Source: three-view drawing plus pictorial views. Frame: mm from the lowest corner of the part. A direction names the side the tool comes from. Give positions to 0.01 mm unless a question says otherwise; leave off trailing zeros. Write each loop counter-clockwise with the first axis right and the second up, starting at its lowest first coordinate (ties: lowest second). Pieces come first, ordered by that corner, then holes.
Q1. Cut plane D-D on x = 16. Return the cut outline in (y, z).
Q2. Line query: L1, parallel to Z at x = 9, y = 2.75; L2, parallel to X at y = 10, z = 4; L3, parallel to Y at x = 12.25, z = 0.5. Output: solid intervals per line, ascending.
Q3. Cut plane B-B on z = 6.25. Return the cut outline in (x, y).
Q4. Reachability of the marked faces 1, 2, 3, 4 and 5 from +Z, -Z, +X, -X, +Y, -Y: full face, straight path, thin tool, end or side. Return the list, or none.
Q5. Cut plane A-A on x = 5. Return the cut outline in (y, z).
Q6. Pin query (flat end, axial travel): pin 1 (6 mm diameter, centred on y = 10.5, z = 2.5, fed in from +X); pin 2 (1 mm diameter, centred on y = 8, z = 7, fed in from -X); pin 3 (5.5 mm diameter, centred on x = 11, y = 7, fed in from +Z). Return the tip coordinate at first contact, or that it passes through.
Q7. Cut plane C-C on y = 10.5. Return the cut outline in (x, z), plus the area to 4 significant figures.
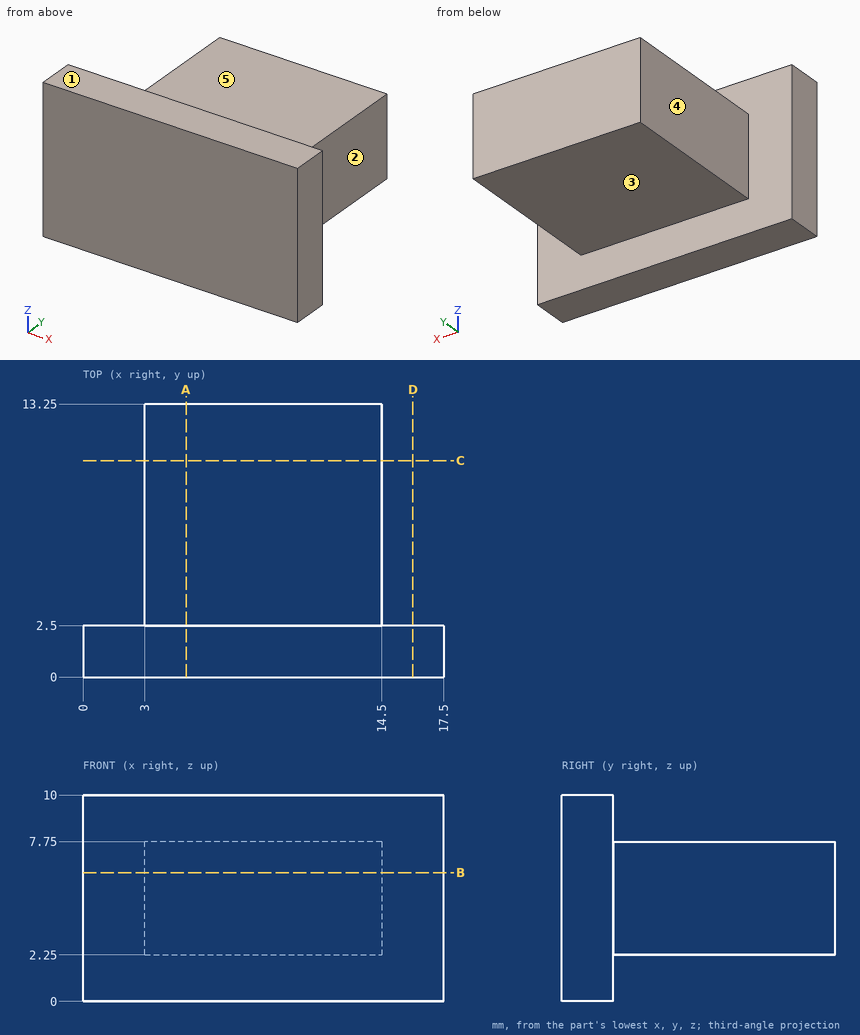
Data:
1. outline: (0, 0) - (2.5, 0) - (2.5, 10) - (0, 10) - close
2. L1: z = 2.25 to 7.75
2. L2: x = 3 to 14.5
2. L3: y = 0 to 2.5
3. outline: (0, 0) - (17.5, 0) - (17.5, 2.5) - (14.5, 2.5) - (14.5, 13.25) - (3, 13.25) - (3, 2.5) - (0, 2.5) - close
4. face 1: +Z, +X, -X, +Y, -Y
4. face 2: +Z, -Z, +X, +Y
4. face 3: -Z, +X, -X, +Y
4. face 4: +Z, -Z, -X, +Y
4. face 5: +Z, +X, -X, +Y
5. outline: (0, 0) - (2.5, 0) - (2.5, 2.25) - (13.25, 2.25) - (13.25, 7.75) - (2.5, 7.75) - (2.5, 10) - (0, 10) - close
6. pin 1: stops at x = 14.5
6. pin 2: stops at x = 3
6. pin 3: stops at z = 7.75
7. outline: (3, 2.25) - (14.5, 2.25) - (14.5, 7.75) - (3, 7.75) - close
7. area: 63.25 mm2
